Build history of the part. All positions in model axes, mm. A direction names the side the tool comes from. Give positions to 0.01 mm unless a question says otherwise; leave off trailing zeros. Order: outer loops, then holes, each group sorted by start corner. A loop starts at its lowest first (then second) coordinate and runs counter-clockwise, first axis right, second up. Notation, with made-up numbers: M 81,13.5 L 86,13.5 A19 ccw 86,22.5 Z; hole C 83,21.5 d4. An arc over 180 degrees is marked long. Use CSV: the item, a comma, the result in double quotes. Start each with the question number.
Item 1: Band-saw the part on A-A on z = -1.7. Give the number of separate pieces and of enclosed holes in the cut face, plus the area to 3 significant figures.
Item 2: Two-plate mould, pull along Y, no slides. Class faces 1 (the flat face through (408, 26.6, -5)), 2 (the flat face through (384, 24, -5.59)): pulls with the +Y half, pulls with the -Y half, needs draft (parallel to the pull), parting line crosses it, or undercut.
Item 3: Which spindle directions (+Z, -Z, +X, -X, +Y, -Y) get a long thin tool onto all of the face, cutting with end or side? Do faces 3 (the flat face through (406.4, 31.5, -3.59)), 4 (the flat face through (408, 35, -5)), 5 (the cylindrical face through (357, 42.6, -4.9)). Say none if no direction does.
Item 4: Band-saw the part on C-C on x = 366. Write the cut outline in (y, z).
Item 5: Pin check, flat tips, straight feed: P1, Ø10, axis at x = 375.5, y = 37.5, coming from the +Z side; P2, Ø3.5, axis at x = 407.5, y = 23, coming from the +Z side; P3, Ø1.8, axis at x = 359, y = 44, coming from the -Z side; P4, Ø8, axis at x = 382.5, y = 31.5, coming from the -Z side. Stop position of each tip, or through.
Item 6: Wall check: line 1 along Y through (x, z) = (400, -1.35); line 2 along X through (y, z) = (38, -3.5); line 3 along X through (y, z) = (45, -1.4). Give the ranges that are in metal, low to high.
from build123d import *

# Parameters (mm, degrees)
BOSS_EXTRUDE1_DEPTH       = 3.59
SHELL1_T                  = 2
CUT_EXTRUDE2_START        = -3.59
SKETCH6_W                 = 26
SKETCH6_H                 = 11.6
CUT_EXTRUDE2_DEPTH        = 417.990251938
CUT_EXTRUDE3_REACH        = 422.58
SKETCH4_R                 = 1.75
BOSS_EXTRUDE2_START       = -0.8
SKETCH4_3_R               = 3
SKETCH4_3_R_2             = 1.75
BOSS_EXTRUDE2_DEPTH       = 4.79
BOSS_EXTRUDE3_START       = -0.41148
SKETCH4_4_R               = 3
SKETCH4_4_R_2             = 1.75
BOSS_EXTRUDE3_DEPTH       = 5.17852
CHAMFER1_SIZE             = 2
CUT_EXTRUDE4_START        = -5.59
CUT_EXTRUDE4_DEPTH        = 2
BOSS_EXTRUDE4_START       = -5.59
BOSS_EXTRUDE4_DEPTH       = 1
BOSS_EXTRUDE5_OUTLINE_R   = 1.508047724
BOSS_EXTRUDE5_DEPTH       = 2.79
BOSS_EXTRUDE5_DRAFT       = 10
BOSS_EXTRUDE5_2_OUTLINE_R = 1.508047724
BOSS_EXTRUDE5_2_DEPTH     = 2.79
BOSS_EXTRUDE5_2_DRAFT     = 10
CUT_EXTRUDE7_START        = -5.59
SKETCH4_5_R               = 3
CUT_EXTRUDE7_DEPTH        = 1.5
FILLET2_R                 = 1


# Read off the part's stored shape, not the designer's step: Boss-Extrude5
with BuildPart() as part:
    # Sketch3 → Boss-Extrude1 (new body)
    # profile 1 of 2: a face of its own
    with BuildSketch(Plane.XY):
        with BuildLine():
            Line((409.499839162, 48.499999974), (360.000160838, 48.499999974))
            ThreePointArc((360.000160838, 48.499999974), (355.756888215, 46.743111785), (354.000000026, 42.499839162))
            Line((354.000000026, 42.499839162), (354.000000026, 15.000161001))
            ThreePointArc((354.000000026, 15.000161001), (355.756887739, 10.756887739), (360.000161001, 9.000000026))
            Line((360.000161001, 9.000000026), (409.499838999, 9.000000026))
            ThreePointArc((409.499838999, 9.000000026), (413.743112261, 10.756887739), (415.499999974, 15.000161001))
            Line((415.499999974, 15.000161001), (415.499999974, 42.499839162))
            ThreePointArc((415.499999974, 42.499839162), (413.743111785, 46.743111785), (409.499839162, 48.499999974))
        make_face()
        with BuildLine():
            ThreePointArc((360, 47.5), (356.46399498, 46.03600502), (355, 42.5))
            Line((355, 42.5), (355, 15))
            ThreePointArc((355, 15), (356.463994503, 11.463994503), (360, 10))
            Line((360, 10), (409.5, 10))
            ThreePointArc((409.5, 10), (413.036005497, 11.463994503), (414.5, 15))
            Line((414.5, 15), (414.5, 42.5))
            ThreePointArc((414.5, 42.5), (413.03600502, 46.03600502), (409.5, 47.5))
            Line((409.5, 47.5), (360, 47.5))
        make_face(mode=Mode.SUBTRACT)
    # profile 2 of 2: a face of its own
    with BuildSketch(Plane.XY):
        with BuildLine():
            Line((409.5, 47.5), (360, 47.5))
            ThreePointArc((360, 47.5), (356.46399498, 46.03600502), (355, 42.5))
            Line((355, 42.5), (355, 15))
            ThreePointArc((355, 15), (356.463994503, 11.463994503), (360, 10))
            Line((360, 10), (409.5, 10))
            ThreePointArc((409.5, 10), (413.036005497, 11.463994503), (414.5, 15))
            Line((414.5, 15), (414.5, 42.5))
            ThreePointArc((414.5, 42.5), (413.03600502, 46.03600502), (409.5, 47.5))
        make_face()
    extrude(amount=-BOSS_EXTRUDE1_DEPTH)

    # Shell1
    shell1_openings = [part.faces().sort_by_distance(p)[0] for p in [
        (384.75, 28.749999938, 0),
    ]]
    offset(amount=SHELL1_T, openings=shell1_openings, kind=Kind.INTERSECTION)

    # Sketch6 → Cut-Extrude2 (cut, through all)
    with BuildSketch(Plane.XY.offset(CUT_EXTRUDE2_START)):
        with Locations((384.62991333, 31.670090703)):
            Rectangle(SKETCH6_W, SKETCH6_H)
    extrude(amount=-CUT_EXTRUDE2_DEPTH, mode=Mode.SUBTRACT)

    # Sketch4 → Cut-Extrude3 (cut, up to next)
    with BuildSketch(Plane.XY, mode=Mode.PRIVATE) as cut_extrude3_sk1:
        with Locations((409.49999888, 42.49999882)):
            Circle(SKETCH4_R)
    cut_extrude3_tool1 = extrude(cut_extrude3_sk1.sketch, amount=-CUT_EXTRUDE3_REACH, mode=Mode.PRIVATE) & part.part
    # Sketch4 → Cut-Extrude3 (cut, up to next)
    with BuildSketch(Plane.XY, mode=Mode.PRIVATE) as cut_extrude3_sk2:
        with Locations((359.99999888, 42.49999882)):
            Circle(SKETCH4_R)
    cut_extrude3_tool2 = extrude(cut_extrude3_sk2.sketch, amount=-CUT_EXTRUDE3_REACH, mode=Mode.PRIVATE) & part.part
    # Sketch4 → Cut-Extrude3 (cut, up to next)
    with BuildSketch(Plane.XY, mode=Mode.PRIVATE) as cut_extrude3_sk3:
        with Locations((359.99999888, 14.99999882)):
            Circle(SKETCH4_R)
    cut_extrude3_tool3 = extrude(cut_extrude3_sk3.sketch, amount=-CUT_EXTRUDE3_REACH, mode=Mode.PRIVATE) & part.part
    # Sketch4 → Cut-Extrude3 (cut, up to next)
    with BuildSketch(Plane.XY, mode=Mode.PRIVATE) as cut_extrude3_sk4:
        with Locations((409.49999888, 14.99999882)):
            Circle(SKETCH4_R)
    cut_extrude3_tool4 = extrude(cut_extrude3_sk4.sketch, amount=-CUT_EXTRUDE3_REACH, mode=Mode.PRIVATE) & part.part
    add(cut_extrude3_tool1.solids().sort_by_distance((409.499999, 42.499999, 0))[0], mode=Mode.SUBTRACT)
    add(cut_extrude3_tool2.solids().sort_by_distance((359.999999, 42.499999, 0))[0], mode=Mode.SUBTRACT)
    add(cut_extrude3_tool3.solids().sort_by_distance((359.999999, 14.999999, 0))[0], mode=Mode.SUBTRACT)
    add(cut_extrude3_tool4.solids().sort_by_distance((409.499999, 14.999999, 0))[0], mode=Mode.SUBTRACT)

    # Sketch4<3> → Boss-Extrude2 (add)
    # profile 1 of 4: a face of its own
    with BuildSketch(Plane.XY.offset(BOSS_EXTRUDE2_START)):
        with Locations((409.49999888, 42.49999882)):
            Circle(SKETCH4_3_R)
        with Locations((409.49999888, 42.49999882)):
            Circle(SKETCH4_3_R_2, mode=Mode.SUBTRACT)
    # profile 2 of 4: a face of its own
    with BuildSketch(Plane.XY.offset(BOSS_EXTRUDE2_START)):
        with Locations((359.99999888, 42.49999882)):
            Circle(SKETCH4_3_R)
        with Locations((359.99999888, 42.49999882)):
            Circle(SKETCH4_3_R_2, mode=Mode.SUBTRACT)
    # profile 3 of 4: a face of its own
    with BuildSketch(Plane.XY.offset(BOSS_EXTRUDE2_START)):
        with Locations((359.99999888, 14.99999882)):
            Circle(SKETCH4_3_R)
        with Locations((359.99999888, 14.99999882)):
            Circle(SKETCH4_3_R_2, mode=Mode.SUBTRACT)
    # profile 4 of 4: a face of its own
    with BuildSketch(Plane.XY.offset(BOSS_EXTRUDE2_START)):
        with Locations((409.49999888, 14.99999882)):
            Circle(SKETCH4_3_R)
        with Locations((409.49999888, 14.99999882)):
            Circle(SKETCH4_3_R_2, mode=Mode.SUBTRACT)
    extrude(amount=-BOSS_EXTRUDE2_DEPTH)

    # Sketch4<4> → Boss-Extrude3 (add)
    # profile 1 of 4: a face of its own
    with BuildSketch(Plane.XY.offset(BOSS_EXTRUDE3_START)):
        with Locations((409.49999888, 42.49999882)):
            Circle(SKETCH4_4_R)
        with Locations((409.49999888, 42.49999882)):
            Circle(SKETCH4_4_R_2, mode=Mode.SUBTRACT)
    # profile 2 of 4: a face of its own
    with BuildSketch(Plane.XY.offset(BOSS_EXTRUDE3_START)):
        with Locations((359.99999888, 42.49999882)):
            Circle(SKETCH4_4_R)
        with Locations((359.99999888, 42.49999882)):
            Circle(SKETCH4_4_R_2, mode=Mode.SUBTRACT)
    # profile 3 of 4: a face of its own
    with BuildSketch(Plane.XY.offset(BOSS_EXTRUDE3_START)):
        with Locations((359.99999888, 14.99999882)):
            Circle(SKETCH4_4_R)
        with Locations((359.99999888, 14.99999882)):
            Circle(SKETCH4_4_R_2, mode=Mode.SUBTRACT)
    # profile 4 of 4: a face of its own
    with BuildSketch(Plane.XY.offset(BOSS_EXTRUDE3_START)):
        with Locations((409.49999888, 14.99999882)):
            Circle(SKETCH4_4_R)
        with Locations((409.49999888, 14.99999882)):
            Circle(SKETCH4_4_R_2, mode=Mode.SUBTRACT)
    extrude(amount=-BOSS_EXTRUDE3_DEPTH)

    # Chamfer1
    chamfer1_edges = [part.edges().sort_by_distance(p)[0] for p in [
        (371.62991333, 31.670090703, -3.59),
        (384.62991333, 37.470090703, -3.59),
        (397.62991333, 31.670090703, -3.59),
        (384.62991333, 25.870090703, -3.59),
    ]]
    chamfer(chamfer1_edges, length=CHAMFER1_SIZE - 0.0001)  # a hair under: the kernel refuses the full size

    # Sketch8 → Cut-Extrude4 (cut)
    with BuildSketch(Plane.XY.offset(CUT_EXTRUDE4_START)):
        Polygon((404.400061047, 26.600064968), (404.400061047, 19.400064968), (411.600061047, 19.400064968), (411.600061047, 21.000064968), (410.000061047, 21.000064968), (408.000061047, 21.000064968), (406.000061047, 21.000064968), (406.000061047, 23.000064968), (406.000061047, 25.000064968), (408.000061047, 25.000064968), (410.000061047, 25.000064968), (411.600061047, 25.000064968), (411.600061047, 26.600064968), align=None)
        Polygon((406.000061047, 33.000064968), (406.000061047, 35.000064968), (408.000061047, 35.000064968), (410.000061047, 35.000064968), (411.600061047, 35.000064968), (411.600061047, 36.600064968), (404.400061047, 36.600064968), (404.400061047, 29.400064968), (411.600061047, 29.400064968), (411.600061047, 31.000064968), (410.000061047, 31.000064968), (408.000061047, 31.000064968), (406.000061047, 31.000064968), align=None)
        Polygon((411.600061047, 35.000064968), (410.000061047, 35.000064968), (410.000061047, 33.000064968), (410.000061047, 31.000064968), (411.600061047, 31.000064968), align=None)
        Polygon((410.000061047, 21.000064968), (411.600061047, 21.000064968), (411.600061047, 25.000064968), (410.000061047, 25.000064968), (410.000061047, 23.000064968), align=None)
    extrude(amount=CUT_EXTRUDE4_DEPTH, mode=Mode.SUBTRACT)


with BuildPart() as cut_extrude4_piece_1:
    # of the separate pieces the step leaves, piece 1, a body of its own (cut_extrude4_pieces)
    add(part.part.solids().sort_by_distance((409.499839162, 48.499999974, -3.59))[0])



with BuildPart() as cut_extrude4_piece_2:
    # of the separate pieces the step leaves, piece 2, a body of its own (cut_extrude4_pieces)
    add(part.part.solids().sort_by_distance((410.000061047, 35.000064968, -3.59))[0])


with BuildPart() as cut_extrude4_piece_3:
    # of the separate pieces the step leaves, piece 3, a body of its own (cut_extrude4_pieces)
    add(part.part.solids().sort_by_distance((406.000061047, 25.000064968, -3.59))[0])


with BuildPart() as cut_extrude4_piece_1_1:
    add(cut_extrude4_piece_1.part)

    add(cut_extrude4_piece_2.part)  # Boss-Extrude4 merges Cut-Extrude4 piece 2

    add(cut_extrude4_piece_3.part)  # Boss-Extrude4 merges Cut-Extrude4 piece 3
    # Sketch8<3> → Boss-Extrude4 (add)
    with BuildSketch(Plane.XY.offset(BOSS_EXTRUDE4_START)):
        Polygon((411.600061047, 35.000064968), (410.000061047, 35.000064968), (410.000061047, 33.000064968), (410.000061047, 31.000064968), (411.600061047, 31.000064968), align=None)
        Polygon((410.000061047, 21.000064968), (411.600061047, 21.000064968), (411.600061047, 25.000064968), (410.000061047, 25.000064968), (410.000061047, 23.000064968), align=None)
    extrude(amount=BOSS_EXTRUDE4_DEPTH)


with BuildPart() as boss_extrude5_tool:
    # Boss-Extrude5 outline → Boss-Extrude5 (with draft: the straight prism first)
    with BuildSketch(Plane.XY.offset(-0.8)):
        with Locations((408.000061047, 33.000064968)):
            Circle(BOSS_EXTRUDE5_OUTLINE_R)
    extrude(amount=-BOSS_EXTRUDE5_DEPTH)
    # Boss-Extrude5: the draft: its side faces are tilted about the plane it starts from
    boss_extrude5_sides = [boss_extrude5_tool.faces().sort_by_distance(p)[0] for p in [
        (406.492013323, 33.000064968, -2.195),
    ]]
    draft(boss_extrude5_sides, Plane.XY.offset(-0.8), BOSS_EXTRUDE5_DRAFT)


with BuildPart() as cut_extrude4_piece_1_2:
    add(cut_extrude4_piece_1_1.part)

    # Boss-Extrude5: add boss_extrude5_tool
    add(boss_extrude5_tool.part)


with BuildPart() as boss_extrude5_2_tool:
    # Boss-Extrude5 2 outline → Boss-Extrude5 2 (with draft: the straight prism first)
    with BuildSketch(Plane.XY.offset(-0.8)):
        with Locations((408.000061047, 23.000064968)):
            Circle(BOSS_EXTRUDE5_2_OUTLINE_R)
    extrude(amount=-BOSS_EXTRUDE5_2_DEPTH)
    # Boss-Extrude5 2: the draft: its side faces are tilted about the plane it starts from
    boss_extrude5_2_sides = [boss_extrude5_2_tool.faces().sort_by_distance(p)[0] for p in [
        (406.492013323, 23.000064968, -2.195),
    ]]
    draft(boss_extrude5_2_sides, Plane.XY.offset(-0.8), BOSS_EXTRUDE5_2_DRAFT)


with BuildPart() as cut_extrude4_piece_1_3:
    add(cut_extrude4_piece_1_2.part)

    # Boss-Extrude5 2: add boss_extrude5_2_tool
    add(boss_extrude5_2_tool.part)

    # Sketch4<5> → Cut-Extrude7 (cut)
    with BuildSketch(Plane.XY.offset(CUT_EXTRUDE7_START)):
        with Locations((409.49999888, 42.49999882)):
            Circle(SKETCH4_5_R)
        with Locations((359.99999888, 42.49999882)):
            Circle(SKETCH4_5_R)
        with Locations((359.99999888, 14.99999882)):
            Circle(SKETCH4_5_R)
        with Locations((409.49999888, 14.99999882)):
            Circle(SKETCH4_5_R)
    extrude(amount=CUT_EXTRUDE7_DEPTH, mode=Mode.SUBTRACT)

    # Fillet2
    fillet2_edges = [cut_extrude4_piece_1_3.edges().sort_by_distance(p)[0] for p in [
        (356.99999888, 14.99999882, -3.59),
        (406.49999888, 42.49999882, -3.59),
        (356.99999888, 42.49999882, -3.59),
        (406.49999888, 14.99999882, -3.59),
    ]]
    fillet(fillet2_edges, radius=FILLET2_R)


solid = cut_extrude4_piece_1_3.part
Model answer:
1,separate pieces,"7"
1,enclosed holes,"5"
1,area,"488 mm^2"
2,face 1,"undercut"
2,face 2,"needs draft"
3,face 3,"+Z"
3,face 4,"+Z, -Z"
3,face 5,"-Z"
4,outline,"M 7,-5.59 L 50.5,-5.59 L 50.5,0 L 48.5,0 L 48.5,-3.59 L 9,-3.59 L 9,0 L 7,0 Z"
5,P1,"stops at z = -3.59"
5,P2,"stops at z = -0.8"
5,P3,"stops at z = -4.09"
5,P4,"passes through"
6,line 1,"y = 7 to 9, 48.5 to 50.5"
6,line 2,"x = 352 to 354, 415.5 to 417.5"
6,line 3,"x = 352.4 to 354.55, 358.34 to 361.66, 407.84 to 411.16, 414.95 to 417.1"
